```python
from build123d import *

# Parameters (mm, degrees)
BOSS_EXTRUDE5_DEPTH      = 40
BOSS_EXTRUDE9_DEPTH      = 10
BOSS_EXTRUDE9_DEPTH_BACK = 50
BOSS_EXTRUDE10_DEPTH     = 120
SKETCH5_R                = 12.5
BOSS_EXTRUDE11_DEPTH     = 127
BOSS_EXTRUDE12_DEPTH     = 127
SKETCH8_W                = 70
SKETCH8_H                = 6
BOSS_EXTRUDE14_DEPTH     = 127
SKETCH9_W                = 70
SKETCH9_H                = 6
BOSS_EXTRUDE15_DEPTH     = 127
SKETCH10_W               = 70
SKETCH10_H               = 6
BOSS_EXTRUDE16_DEPTH     = 124
EXTRUDE_THIN1_DEPTH      = 5


with BuildPart() as part:
    # Sketch1 → Boss-Extrude5 (new body)
    with BuildSketch(Plane(origin=(0, 0, 0), x_dir=(1, 0, 0), z_dir=(0, 1, 0))):
        Polygon((-140.670056302, -135.044197431), (46.616677458, -189.345941025), (187.28673376, -54.301743594), (140.670056302, 135.044197431), (-46.616677458, 189.345941025), (-187.28673376, 54.301743594), align=None)
        Polygon((165.106211473, -47.870743331), (124.010385559, 119.050801792), (-41.095825913, 166.921545124), (-165.106211473, 47.870743331), (-124.010385559, -119.050801792), (41.095825913, -166.921545124), align=None, mode=Mode.SUBTRACT)
    extrude(amount=BOSS_EXTRUDE5_DEPTH)



with BuildPart() as body_2:
    # Sketch3 → Boss-Extrude9 (new body, two sides)
    with BuildSketch(Plane.XZ) as boss_extrude9_sk:
        with BuildLine():
            Line((3.733551148, -26.665719488), (-15.686545368, -21.8845218))
            ThreePointArc((-15.686545368, -21.8845218), (-33.985168902, 8.367095954), (-3.733551148, 26.665719488))
            Line((-3.733551148, 26.665719488), (15.686545368, 21.8845218))
            ThreePointArc((15.686545368, 21.8845218), (33.985168902, -8.367095954), (3.733551148, -26.665719488))
        make_face()
        with BuildLine():
            Line((6.124149992, -16.955671231), (-13.295946524, -12.174473543))
            ThreePointArc((-13.295946524, -12.174473543), (-24.275120644, 5.97649711), (-6.124149992, 16.955671231))
            Line((-6.124149992, 16.955671231), (13.295946524, 12.174473543))
            ThreePointArc((13.295946524, 12.174473543), (24.275120644, -5.97649711), (6.124149992, -16.955671231))
        make_face(mode=Mode.SUBTRACT)
    extrude(amount=BOSS_EXTRUDE9_DEPTH)
    extrude(boss_extrude9_sk.sketch, amount=-BOSS_EXTRUDE9_DEPTH_BACK)


with BuildPart() as part_1:
    add(part.part)

    add(body_2.part)  # Boss-Extrude10 merges body 2
    # Sketch4 → Boss-Extrude10 (add)
    with BuildSketch(Plane(origin=(-144.558298516, 0, 35.590029231), x_dir=(-0.239059884, 0, -0.971004826), z_dir=(0.971004826, 0, -0.239059884))):
        with BuildLine():
            ThreePointArc((12.5, 20), (0, 32.5), (-12.5, 20))
            Line((-12.5, 20), (12.5, 20))
        make_face()
        with BuildLine():
            Line((12.5, 20), (-12.5, 20))
            ThreePointArc((-12.5, 20), (0, 7.5), (12.5, 20))
        make_face()
    extrude(amount=BOSS_EXTRUDE10_DEPTH)

    # Sketch5 → Boss-Extrude11 (add)
    with BuildSketch(Plane(origin=(41.457279823, 0, -142.986173458), x_dir=(0.960444789, 0, 0.27847048), z_dir=(-0.27847048, 0, 0.960444789))):
        with Locations((0, 20)):
            Circle(SKETCH5_R)
    extrude(amount=BOSS_EXTRUDE11_DEPTH)

    # Sketch6 → Boss-Extrude12 (add)
    with BuildSketch(Plane(origin=(103.101018693, 0, 107.396144227), x_dir=(-0.721384904, 0, 0.692534346), z_dir=(-0.692534346, 0, -0.721384904))):
        with BuildLine():
            ThreePointArc((-12.5, 20), (0, 7.5), (12.5, 20))
            Line((12.5, 20), (-12.5, 20))
        make_face()
        with BuildLine():
            Line((-12.5, 20), (12.5, 20))
            ThreePointArc((12.5, 20), (0, 32.5), (-12.5, 20))
        make_face()
    extrude(amount=BOSS_EXTRUDE12_DEPTH)

    # Sketch8 → Boss-Extrude14 (add)
    with BuildSketch(Plane(origin=(-103.101018693, 0, -107.396144227), x_dir=(0.721384904, 0, -0.692534346), z_dir=(0.692534346, 0, 0.721384904))):
        with Locations((0, 37)):
            Rectangle(SKETCH8_W, SKETCH8_H)
    extrude(amount=BOSS_EXTRUDE14_DEPTH)

    # Sketch9 → Boss-Extrude15 (add)
    with BuildSketch(Plane(origin=(-41.457279823, 0, 142.986173458), x_dir=(-0.960444789, 0, -0.27847048), z_dir=(0.27847048, 0, -0.960444789))):
        with Locations((0, 37)):
            Rectangle(SKETCH9_W, SKETCH9_H)
    extrude(amount=BOSS_EXTRUDE15_DEPTH)

    # Sketch10 → Boss-Extrude16 (add)
    with BuildSketch(Plane(origin=(144.558298516, 0, -35.590029231), x_dir=(0.239059884, 0, 0.971004826), z_dir=(-0.971004826, 0, 0.239059884))):
        with Locations((0, 37)):
            Rectangle(SKETCH10_W, SKETCH10_H)
    extrude(amount=BOSS_EXTRUDE16_DEPTH)

    # Sketch14 → Extrude-Thin1 (add)
    with BuildSketch(Plane(origin=(0, 40, 0), x_dir=(1, 0, 0), z_dir=(0, 1, 0))):
        Polygon((50.306594431, -0.487856845), (64.871666817, 3.098041421), (58.895169707, 27.373162065), (44.330097321, 23.787263799), (46.720696165, 14.077215541), (51.575720293, 15.272514963), (52.771019715, 10.417490835), (47.915995587, 9.222191413), align=None)
        Polygon((-25.575793637, -43.322860332), (-29.752850836, -57.72953216), (-5.741731123, -64.691294159), (-1.564673924, -50.284622331), (-11.169121809, -47.499917532), (-12.561474209, -52.302141474), (-17.363698151, -50.909789074), (-15.971345751, -46.107565132), align=None)
        Polygon((-24.730800794, 43.810717177), (-35.118815981, 54.631490739), (-53.153438584, 37.318132094), (-42.765423397, 26.497358532), (-35.551574356, 33.42270199), (-39.014246085, 37.029626511), (-35.407321564, 40.49229824), (-31.944649835, 36.885373719), align=None)
    extrude(amount=EXTRUDE_THIN1_DEPTH)


solid = part_1.part
```
Design review of the part built by this model. Coordinates are the model's own, in mm. A direction names the side the tool comes from. Give positions to 0.01 mm unless a question says otherwise; leave off trailing zeros. Write each loop counter-clockwise with the first axis right and the second up, starting at its lowest first coordinate (ties: lowest second). Pieces come first, ordered by that corner, then holes. Notation, with made-up numbers: (63.25, 14.5) - (68.25, 14.5) arc R14 ccw to (68.25, 26.5) - close; hole circle Ø2 at (-5, -36). An arc over 180 degrees is marked (long way). Return JSON: item names as keys, results as strings. Group by question number.
(1) We need section A-A, the plane z = 124. Give the boundary of the cut face in (x, y), then the cut area to 3 significant figures.
(2) We need section B-B, the plane z = -160. Give the boundary of the cut face in (x, y), then the cut area to 3 significant figures.
(3) To check wall thickness, follow probe 1 along X at (y, z) = (13, 89.5); probe 2 along X at (y, z) = (21.5, 98); probe 3 along Y at (x, z) = (-141, 115). State the ranges of each line that lie inside material, in increasing order.
(4) Insertion check: pin 1 (23.5 mm diameter, centred on x = -13.5, z = 55.5, fed in from +Y); pin 2 (8 mm diameter, centred on x = 58.5, y = 24, fed in from -Z); pin 3 (8 mm diameter, centred on x = -96, y = 8, fed in from +Z). Each pin has a flat end and moves straight along its axis. Give the tip position at first contact, or say it passes through.
(5) Mouldability with a two-part tool opening along X and no side actions: class faces 1 (the flat face through (1.728, 37.042, -31.982)), 2 (the flat face through (0, 50, -18)), 3 (the flat face through (164.305, 19.72, -39.046)) as +X half, -X half, draft (parallel to the pull), parting line (faces both ways), or undercut.
(6) We need section C-C, the plane x = -106. Give the number of separate pieces and of enclosed holes in the cut face, then the cut area to 3 significant figures.
(7) Machinability: for faces 4 (the flat face through (-102.23, 19.72, -108.23)), 5 (the flat face through (54, 45, -14)), 6 (the flat face through (-5, 40, 30)), which of the approach directions +Z, -Z, +X, -X, +Y, -Y give a long, thin tool a straight path to every point of the face, cutting with its end or side? Answer none if there is none.
Reported:
{
 "1": {"outline": "(-143.39, 0) - (-106.94, 0) - (-106.94, 40) - (-143.39, 40) - close; (-72.39, 34) - (0.49, 34) - (0.49, 40) - (-72.39, 40) - close; (85.81, 0) - (114.68, 0) - (114.68, 40) - (85.81, 40) - close", "area": "3,050 mm2"},
 "2": {"outline": "(-77.19, 0) - (-48.31, 0) - (-48.31, 40) - (-77.19, 40) - close; (-17.22, 0) - (54.6, 0) - (54.6, 40) - (-17.22, 40) - close", "area": "4,030 mm2"},
 "3": {"probe 1": "x = -151.88 to -131.29, 71.56 to 100.28, 121.74 to 150.62", "probe 2": "x = -149.79 to -129.19, 76.88 to 111.28, 112.89 to 141.77", "probe 3": "y = 0 to 40"},
 "4": {"pin 1": "stops at y = 45", "pin 2": "stops at z = -160.03", "pin 3": "stops at z = 149.16"},
 "5": {"face 1": "undercut", "face 2": "draft", "face 3": "+X half"},
 "6": {"separate pieces": "3", "enclosed holes": "0", "area": "2,720 mm2"},
 "7": {"face 4": "-Y", "face 5": "+Z, -Z, +X, +Y", "face 6": "+Y"}
}
